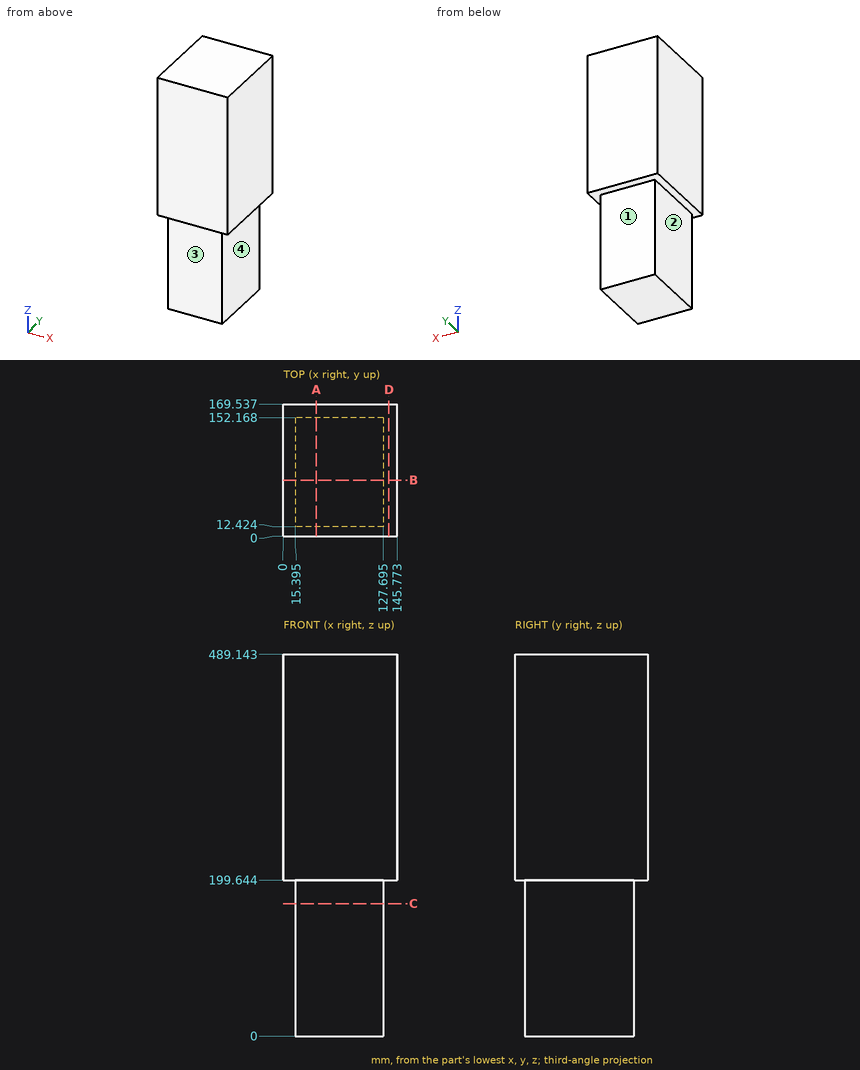
Part print with two shaded views. Sizes in mm from the minimum x, y, z corner. A direction names the side the tool comes from. Round coordinates to 2 decimals unless told otherwise and drop trailing zeros. Order: outer loops, then holes, each group sorted by start corner. A loop starts at its lowest first (then second) coordinate and runs counter-clockwise, first axis right, second up. Notation, with made-up numbers: (-3, -22) - (31, -22) arc R25 cw to (31, 8) - close; hole circle Ø3 at (67, 73.25). An arc over 180 degrees is marked (long way). Return JSON: item names as keys, results as strings.
(1) Cut at C-C (z = 169.5). Give the cut face in (x, y) (1 decimal), then the cut area to 3 significant figures.
Answer key:
{"outline": "(15.4, 12.4) - (127.7, 12.4) - (127.7, 152.2) - (15.4, 152.2) - close", "area": "15,700 mm^2"}
(2) Cut at D-D (x = 135). Give the cut face in (y, z).
Answer key:
{"outline": "(0, 199.64) - (169.54, 199.64) - (169.54, 489.14) - (0, 489.14) - close"}
(3) Pin check, flat tips, straight feed: pin 1 Ø1.5 at (y, z) = (89, 52.5) entering from +X (1 decimal); pin 2 Ø8 at (y, z) = (146, 339) entering from -X; pin 3 Ø8 at (x, z) = (41.5, 131) entering from -Y; pin 4 Ø4 at (x, z) = (87.5, 162.5) entering from +Y. Stop position of each tip, or through.
Answer key:
{"pin 1": "stops at x = 127.7", "pin 2": "stops at x = 0", "pin 3": "stops at y = 12.42", "pin 4": "stops at y = 152.17"}
(4) Wall check: probe 1 along Z at (x, y) = (135.5, 31); probe 2 along X at (y, z) = (19, 164.5) (1 decimal); probe 3 along Y at (x, z) = (100, 89.5). Give the ranges that are in metal, low to high. Write a range as from..to.
Answer key:
{"probe 1": "z = 199.64..489.14", "probe 2": "x = 15.4..127.7", "probe 3": "y = 12.42..152.17"}
(5) Tool access for the marked faces 1, 2, 3 and 4: list every direction of +Z, -Z, +X, -X, +Y, -Y with a clear straight run to the whole face (end or side of a thin tool).
Answer key:
{"face 1": "-Z, +X, -X, +Y", "face 2": "-Z, -X, +Y, -Y", "face 3": "-Z, +X, -X, -Y", "face 4": "-Z, +X, +Y, -Y"}
(6) Cut at A-A (x = 42). Give the cut face in (y, z), then the cut area to 3 significant figures.
Answer key:
{"outline": "(0, 199.64) - (12.42, 199.64) - (12.42, 0) - (152.17, 0) - (152.17, 199.64) - (169.54, 199.64) - (169.54, 489.14) - (0, 489.14) - close", "area": "77,000 mm^2"}
(7) Cut at B-B (y = 72). Give the cut face in (x, z) (1 decimal).
Answer key:
{"outline": "(0, 199.6) - (15.4, 199.6) - (15.4, 0) - (127.7, 0) - (127.7, 199.6) - (145.8, 199.6) - (145.8, 489.1) - (0, 489.1) - close"}
